Work out the finished part from the listing and answer in its coordinate system (mm). A direction names the side the tool comes from. Coordinates: 2 decimals unless noted, no trailing zeros. Order: outer loops, then holes, each group sorted by start corner. A loop starts at its lowest first (then second) coordinate and runs counter-clockwise, first axis right, second up. Notation, with made-up numbers: (82.25, -8.5) - (138.25, -8.5) arc R16 cw to (138.25, 22.5) - close; hole circle Ø7 at (1, 7.5). An arc over 180 degrees is marked (long way). Use CSV: the item, a comma, the result in double quotes. Start each with the question number.
Autodesk Inventor part; units mm, degrees
ref_plane "YZ Plane" through (0, 0, 0) normal (1, 0, 0) x (0, 1, 0)
ref_plane "XZ Plane" through (0, 0, 0) normal (0, 1, 0) x (-1, 0, 0)
ref_plane "XY Plane" through (0, 0, 0) normal (0, 0, 1) x (1, 0, 0)
sketch "Sketch1" plane through (0, 0, 0) normal (0, 0, 1) x (1, 0, 0)
  line L0 (0, 0) -> (76.2, 0)
  arc A0 (0, 0) -> (0, -38.1) centre (0, -19.05) ccw
  arc A1 (76.2, -38.1) -> (76.2, 0) centre (76.2, -19.05) ccw
  line L1 (76.2, -38.1) -> (63.5, -38.1)
  line L2 (0, -38.1) -> (12.7, -38.1)
  arc A2 (21.5833, -46.9837) -> (12.7, -38.1) centre (12.7, -46.9833) ccw
  arc A3 (21.5833, -46.9837) -> (22.9529, -55.026) centre (45.8763, -46.9845) ccw
  arc A4 (22.9529, -55.026) -> (25.9489, -57.15) centre (25.9489, -53.975) ccw
  arc A5 (63.5, -38.1) -> (54.6167, -46.9837) centre (63.5, -46.9833) ccw
  arc A6 (53.2471, -55.026) -> (54.6167, -46.9837) centre (30.3237, -46.9845) ccw
  arc A7 (50.2511, -57.15) -> (53.2471, -55.026) centre (50.2511, -53.975) ccw
  line L3 (25.9489, -57.15) -> (50.2511, -57.15)
  circle A8 centre (0, -19.05) radius 1.778
  circle A9 centre (76.2, -19.05) radius 1.778
  circle A10 centre (38.1, -46.9845) radius 1.778
  line L4 (-19.05, -19.05) -> (-19.05, 0)
  line L5 (95.25, -19.05) -> (95.25, 0)
  point P0 (23.8125, -57.15)
  dimension "d0" = 76.2
  dimension "d1" = 38.1
  dimension "d5" = 12.7
  dimension "d6" = 12.7
  dimension "d8" = 3.175
  dimension "d9" = 3.556
  dimension "d10" = 3.556
  dimension "d11" = 3.556
  dimension "d14" = 19.05
  dimension "d15" = 19.05
extrude "Extrusion1" add sketch "Sketch1" along normal blind 5.842
properties part number "casing"
1) The part is cut by section D-D on y = -50.5. Determine the outline of the cut face in (x, z), plus the area to 3 significant figures.
2) Straight lines are drawn through the part: line 1 (Y direction, x = 38.1, z = 3.35); line 2 (X direction, y = -18, z = 1.3); line 3 (X direction, y = -20.5, z = 0.95). For each, find the intervals that lie inside material, in ascending order. Write a range as [from, to].
3) Flat-ended cylindrical pins translate along their axes: P1, Ø5, axis at x = 7, y = -31.5, coming from the -Z side; P2, Ø3, axis at x = 64, z = 2, coming from the -Y side; P3, Ø1, axis at x = 78, z = 2, coming from the -Y side. Find the tip coordinate at first contact, or state that the pin passes through.
4) The part is cut by section A-A on y = -19.05. Determine the outline of the cut face in (x, z), plus the area to 3 significant figures.
5) For faces 4 (the face through (6, -38.1, 3)), 5 (the face through (70, -38.1, 3)), 6 (the face through (38, -57.15, 3)), determine the directions among +Z, -Z, +X, -X, +Y, -Y from which every point of the face is accessible in a straight line to the end or side of a thin tool.
6) The part is cut by section B-B on x = 38.1. Determine the outline of the cut face in (y, z).
7) The part is cut by section C-C on z = 3.65. State how many separate pieces and enclosed holes the cut face has, plus the area to 3 significant figures.
8) For a pull along Y with two mould halves and no side action, classify faces 1 (the face through (77.156, -20.549, 2.88)), 2 (the face through (-19.045, -19.469, 2.88)), 3 (the face through (18.91, -40.63, 2.88)) as +Y half, -Y half, draft (parallel to the pull), parting line (faces both ways), or undercut.
Answer key:
1,outline,"(21.84, 0) - (54.36, 0) - (54.36, 5.84) - (21.84, 5.84) - close"
1,area,"190 mm^2"
2,line 1,"[-57.15, -48.76], [-45.21, 0]"
2,line 2,"[-19.02, -1.43], [1.43, 74.77], [77.63, 95.22]"
2,line 3,"[-18.99, -1.03], [1.03, 75.17], [77.23, 95.19]"
3,P1,"z = 0"
3,P2,"y = -38.16"
3,P3,"y = -38.06"
4,outline,"(-19.05, 0) - (-1.78, 0) - (-1.78, 5.84) - (-19.05, 5.84) - close; (1.78, 0) - (74.42, 0) - (74.42, 5.84) - (1.78, 5.84) - close; (77.98, 0) - (95.25, 0) - (95.25, 5.84) - (77.98, 5.84) - close"
4,area,"626 mm^2"
5,face 4,"+Z, -Z, -X, -Y"
5,face 5,"+Z, -Z, +X, -Y"
5,face 6,"+Z, -Z, +X, -X, -Y"
6,outline,"(-57.15, 0) - (-48.76, 0) - (-48.76, 5.84) - (-57.15, 5.84) - close; (-45.21, 0) - (0, 0) - (0, 5.84) - (-45.21, 5.84) - close"
7,separate pieces,"1"
7,enclosed holes,"3"
7,area,"4,660 mm^2"
8,face 1,"undercut"
8,face 2,"parting line"
8,face 3,"-Y half"
